Autodesk Inventor part; units mm, degrees
ref_plane "Plano de trabajo1" through (0, 0, 6) normal (0, 0, 1) x (1, 0, 0)
ref_plane "YZ Plane" through (0, 0, 0) normal (1, 0, 0) x (0, 1, 0)
ref_plane "XZ Plane" through (0, 0, 0) normal (0, 1, 0) x (-1, 0, 0)
sketch "Boceto1" plane through (0, 0, 0) normal (0, 0, 1) x (1, 0, 0)
  line L0 (-0.9, -2.4) -> (0.9, -2.4)
  line L1 (0.9, -2.4) -> (0.9, 2.4)
  line L2 (0.9, 2.4) -> (-0.9, 2.4)
  line L3 (-0.9, 2.4) -> (-0.9, -2.4)
  line L4 (-0.9, -2.4) -> (0.9, 2.4) construction
  line L5 (0.9, -2.4) -> (-0.9, 2.4) construction
  line L6 (2.4, -0.9) -> (-2.4, -0.9)
  line L7 (-2.4, -0.9) -> (-2.4, 0.9)
  line L8 (-2.4, 0.9) -> (2.4, 0.9)
  line L9 (2.4, 0.9) -> (2.4, -0.9)
  line L10 (2.4, -0.9) -> (-2.4, 0.9) construction
  line L11 (-2.4, -0.9) -> (2.4, 0.9) construction
  circle A0 centre (0, 0) radius 1.45
  point P0 (1.1369, 0.9)
  point P1 (0.9, 1.1369)
  point P2 (-0.9, 1.1369)
  point P3 (-1.1369, 0.9)
  point P4 (-1.1369, -0.9)
  point P5 (-0.9, -1.1369)
  point P6 (0.9, -1.1369)
  point P7 (1.1369, -0.9)
  dimension "d14" = 2.9
  dimension "d15" = 1.8
  dimension "d16" = 4.8
extrude "Extrusión1" add sketch "Boceto1" along normal blind 13.31
ref_plane "Plano de trabajo1" through (0, 0, 6) normal (0, 0, 1) x (1, 0, 0)
sketch "Boceto2" plane through (0, 0, 6) normal (0, 0, 1) x (1, 0, 0)
  line L0 (2.4, 0.9) -> (1.1369, 0.9) construction
  circle A0 centre (0, 0) radius 2.5632
extrude "Extrusión2" add sketch "Boceto2" along normal blind 3
properties part number "EjeCortoGrua"
Model file for the job. Use its own axes, mm. A direction names the side the tool comes from. Coordinates: 2 decimals unless noted, no trailing zeros. Write each loop counter-clockwise with the first axis right and the second up, starting at its lowest first coordinate (ties: lowest second). Pieces come first, ordered by that corner, then holes. Notation, with made-up numbers: (44.5, -2) - (95.5, -2) arc R30 cw to (95.5, 35) - close; hole circle Ø2 at (-8.75, 51). An arc over 180 degrees is marked (long way). Use a Markdown table: item, result. Add a question column.
Item 1: Band-saw the part on D-D, the plane z = 6.25. Write the cut outline in (x, y).
Item 2: Band-saw the part on A-A, the plane z = 11. Write the cut outline in (x, y).
Item 3: Drop flat-ended pins along their axis: pin 1 (0.9 mm diameter, centred on x = 0.5, z = 4, fed in from +Y); pin 2 (1.4 mm diameter, centred on y = 0.5, z = 2, fed in from +X); pin 3 (0.6 mm diameter, centred on y = -2, z = 11, fed in from -X). Give the stop position or say it passes through.
Item 4: Drill centre lines: line 1 along X through (y, z) = (-2.1, 0.75); line 2 along X through (y, z) = (-0.75, 2.5); line 3 along Z through (x, y) = (-1.1, 1.85). Where is each one in solid material? Low to high.
Item 5: Band-saw the part on B-B, the plane y = 0. Write the cut outline in (x, z), and give its area (3 significant figures).
Item 6: 3-axis set-ups, long thin cutter, end or side, ignore diameter. For faces 1 (the face through (0, -2.4, 11)), 2 (the face through (2, 0.9, 11)), 3 (the face through (-1.5, 1.5, 6)): which of +Z, -Z, +X, -X, +Y, -Y reach the whole face in a straight line?
A:
| question | item | result |
|---|---|---|
| 1 | outline | circle Ø5.13 at (0, 0) |
| 2 | outline | (-2.4, -0.9) - (-1.14, -0.9) arc R1.45 ccw to (-0.9, -1.14) - (-0.9, -2.4) - (0.9, -2.4) - (0.9, -1.14) arc R1.45 ccw to (1.14, -0.9) - (2.4, -0.9) - (2.4, 0.9) - (1.14, 0.9) arc R1.45 ccw to (0.9, 1.14) - (0.9, 2.4) - (-0.9, 2.4) - (-0.9, 1.14) arc R1.45 ccw to (-1.14, 0.9) - (-2.4, 0.9) - close |
| 3 | pin 1 | stops at y = 2.4 |
| 3 | pin 2 | stops at x = 2.4 |
| 3 | pin 3 | stops at x = -0.9 |
| 4 | line 1 | x = -0.9 to 0.9 |
| 4 | line 2 | x = -2.4 to 2.4 |
| 4 | line 3 | z = 6 to 9 |
| 5 | outline | (-2.56, 6) - (-2.4, 6) - (-2.4, 0) - (2.4, 0) - (2.4, 6) - (2.56, 6) - (2.56, 9) - (2.4, 9) - (2.4, 13.31) - (-2.4, 13.31) - (-2.4, 9) - (-2.56, 9) - close |
| 5 | area | 64.9 mm² |
| 6 | face 1 | +Z, +X, -X, -Y |
| 6 | face 2 | +Z, +X, +Y |
| 6 | face 3 | -Z, -X, +Y |
